Geometry: see drawing. Coordinates: mm, zero at the bounding-box minimum. Round coordinates to 2 decimals unless told otherwise and drop trailing zeros. Loops run counter-clockwise (first coordinate to the right, second up) from the corner with the lowest first, then second, coordinate; pieces in that order, holes last. Notation, with made-up numbers: (-10.5, 43.5) - (22.5, 43.5) arc R9 ccw to (22.5, 53.5) - close; hole circle Ø8 at (75.25, 26.5). An arc over 180 degrees is marked (long way). Write item = value, one per line. Start each with the question number.
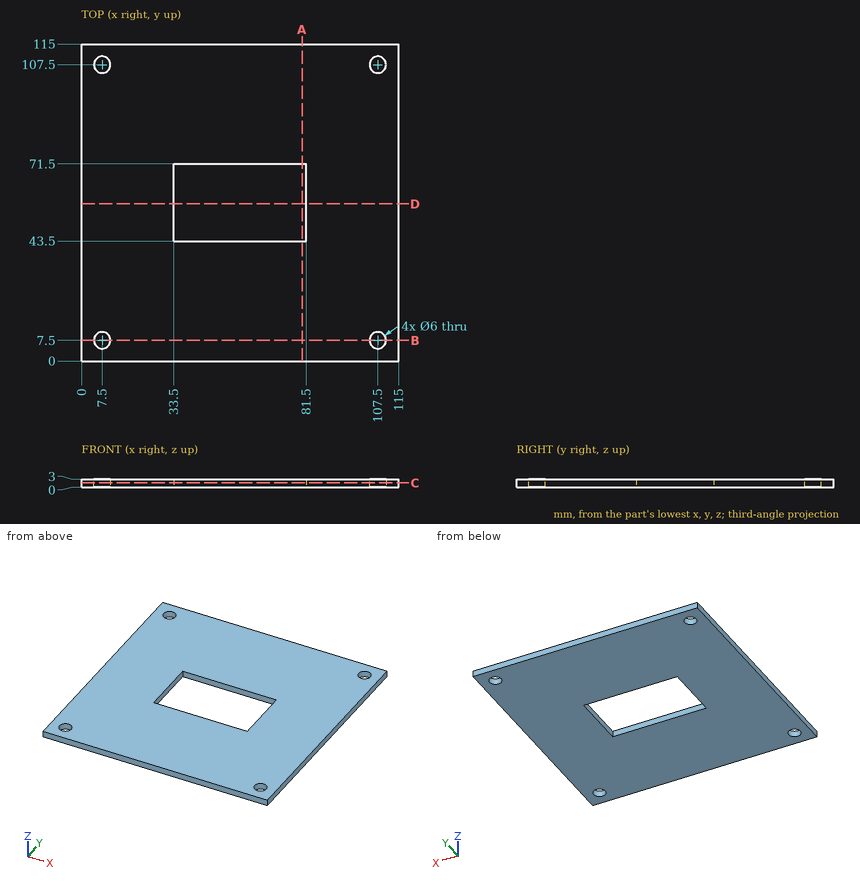
(1) Material intervals for line 1 along Y through (x, z) = (107.5, 2.25); line 2 along Y through (x, z) = (55, 1); line 3 along X through (y, z) = (58, 0.75), sorted ascending. Write a range as from..to.
(2) Cut plane B-B (y = 7.5). Output: boundary loops of the cut face in (x, z).
(3) Cut plane D-D (y = 57). Output: boundary loops of the cut face in (x, z).
(4) Cut plane C-C (z = 1.6). Output: boundary loops of the cut face in (x, y), and give its area (3 significant figures).
(5) Cut plane A-A (x = 80). Output: boundary loops of the cut face in (y, z), and give its area (3 significant figures).
Solution:
q1.line_1 = 0..4.5, 10.5..104.5, 110.5..115
q1.line_2 = 0..43.5, 71.5..115
q1.line_3 = 0..33.5, 81.5..115
q2.outline = (0, 0) - (4.5, 0) - (4.5, 3) - (0, 3) - close; (10.5, 0) - (104.5, 0) - (104.5, 3) - (10.5, 3) - close; (110.5, 0) - (115, 0) - (115, 3) - (110.5, 3) - close
q3.outline = (0, 0) - (33.5, 0) - (33.5, 3) - (0, 3) - close; (81.5, 0) - (115, 0) - (115, 3) - (81.5, 3) - close
q4.outline = (0, 0) - (115, 0) - (115, 115) - (0, 115) - close; hole circle Ø6 at (7.5, 7.5); hole circle Ø6 at (7.5, 107.5); hole (33.5, 43.5) - (81.5, 43.5) - (81.5, 71.5) - (33.5, 71.5) - close; hole circle Ø6 at (107.5, 7.5); hole circle Ø6 at (107.5, 107.5)
q4.area = 11,800 mm^2
q5.outline = (0, 0) - (43.5, 0) - (43.5, 3) - (0, 3) - close; (71.5, 0) - (115, 0) - (115, 3) - (71.5, 3) - close
q5.area = 261 mm^2
